```python
from build123d import *

# Parameters (mm, degrees)
F2_DEPTH = 10
F4_DEPTH = 10
F5_W     = 50
F5_H     = 6.6666666667
F6_DEPTH = 15


with BuildPart() as f2:
    # F1 (on Front) → F2 (new body, symmetric)
    with BuildSketch(Plane.XZ):
        Polygon((450, -75), (600, 75), (-600, 75), (-450, -75), align=None)
    extrude(amount=F2_DEPTH, both=True)

    # F3 (on Front) → F4 (cut, symmetric)
    with BuildSketch(Plane.XZ):
        Polygon((-541.7157287525, 45), (-555.8578643763, 30.8578643763), (-525.8578643763, 0.8578643763), (-511.7157287525, 15), align=None)
        Polygon((-451.7157287525, -45), (-481.7157287525, -15), (-495.8578643763, -29.1421356237), (-465.8578643763, -59.1421356237), align=None)
        Polygon((525.8578643763, 0.8578643763), (555.8578643763, 30.8578643763), (541.7157287525, 45), (511.7157287525, 15), align=None)
        Polygon((495.8578643763, -29.1421356237), (481.7157287525, -15), (451.7157287525, -45), (465.8578643763, -59.1421356237), align=None)
    extrude(amount=F4_DEPTH, both=True, mode=Mode.SUBTRACT)

    # F5 (on face) → F6 (join)
    with BuildSketch(Plane.XZ.offset(10)):
        with Locations((0, -65)):
            Rectangle(F5_W, F5_H)
        with Locations((200, -65)):
            Rectangle(F5_W, F5_H)
        with Locations((400, -65)):
            Rectangle(F5_W, F5_H)
        with Locations((-200, -65)):
            Rectangle(F5_W, F5_H)
        with Locations((-400, -65)):
            Rectangle(F5_W, F5_H)
    extrude(amount=F6_DEPTH)


solid = f2.part
```
Design review of the part built by this model. Coordinates are the model's own, in mm. A direction names the side the tool comes from. Give positions to 0.01 mm unless a question says otherwise; leave off trailing zeros. Order: outer loops, then holes, each group sorted by start corner. A loop starts at its lowest first (then second) coordinate and runs counter-clockwise, first axis right, second up. Notation, with made-up numbers: (37, 78.5) - (62, 78.5) arc R16 cw to (62, 103.5) - close; hole circle Ø4 at (4, -9). An arc over 180 degrees is marked (long way). Use a Markdown table: item, result. Add a question column.
(1) Add section A-A on y = -4. Give the boundary of the cut face in (x, z), then the cut area to 3 significant figures.
(2) Mouldability with a two-part tool opening along X and no side actions: class faces 3 (the face through (511, 0, -14)), 4 (the face through (-578, 0, 53)), 5 (the face through (-526.506, 0.14, 29.79)), 6 (the face through (-8, 10, 1)) as +X half, -X half, draft (parallel to the pull), parting line (faces both ways), or undercut.
(3) Machinability: for faces 1 (the face through (-511, 0, -14)), 2 (the face through (526.926, 0.14, 30.21)), which of the approach directions +Z, -Z, +X, -X, +Y, -Y give a long, thin tool a straight path to every point of the face, cutting with its end or side? Answer none if there is none.
(4) Wall thickness on probe 1 along X at (y, z) = (2.5, 15); probe 2 along Y at (x, z) = (390, 61.5); probe 3 along Z at (x, y) = (-464, -2): over which ranges is each line inside the solid? List them lowest first. Write a range as [from, to].
(5) Clearance check with flat-ended pins moving along their axes: P1, Ø5, axis at x = 291.5, y = -14.5, coming from the +Z side; P2, Ø3.5, axis at y = -19.5, z = -63.5, coming from the -X side; P3, Ø12, axis at x = -399, y = -18.5, coming from the +Z side; P4, Ø7.5, axis at y = -16, z = -66, coming from the +X side. State where each tip first meets the part, or that it passes through.
(6) Add section B-B on x = -4. Give the boundary of the cut face in (y, z), then the cut area to 3 significant figures.
(7) Add section C-C on x = -141.5. Give the boundary of the cut face in (y, z).
Report:
| question | item | result |
|---|---|---|
| 1 | outline | (-600, 75) - (-555.86, 30.86) - (-541.72, 45) - (-511.72, 15) - (-525.86, 0.86) - (-495.86, -29.14) - (-481.72, -15) - (-451.72, -45) - (-465.86, -59.14) - (-450, -75) - (450, -75) - (465.86, -59.14) - (451.72, -45) - (481.72, -15) - (495.86, -29.14) - (525.86, 0.86) - (511.72, 15) - (541.72, 45) - (555.86, 30.86) - (600, 75) - close |
| 1 | area | 154,000 mm² |
| 2 | face 3 | +X half |
| 2 | face 4 | -X half |
| 2 | face 5 | undercut |
| 2 | face 6 | draft |
| 3 | face 1 | -Z, -X, +Y, -Y |
| 3 | face 2 | +Y, -Y |
| 4 | probe 1 | x = [-511.72, 511.72] |
| 4 | probe 2 | y = [-10, 10] |
| 4 | probe 3 | z = [-61, -57.28], [-32.72, 75] |
| 5 | P1 | passes through |
| 5 | P2 | stops at x = -425 |
| 5 | P3 | stops at z = -61.67 |
| 5 | P4 | stops at x = 425 |
| 6 | outline | (-25, -68.33) - (-10, -68.33) - (-10, -75) - (10, -75) - (10, 75) - (-10, 75) - (-10, -61.67) - (-25, -61.67) - close |
| 6 | area | 3,100 mm² |
| 7 | outline | (-10, -75) - (10, -75) - (10, 75) - (-10, 75) - close |
